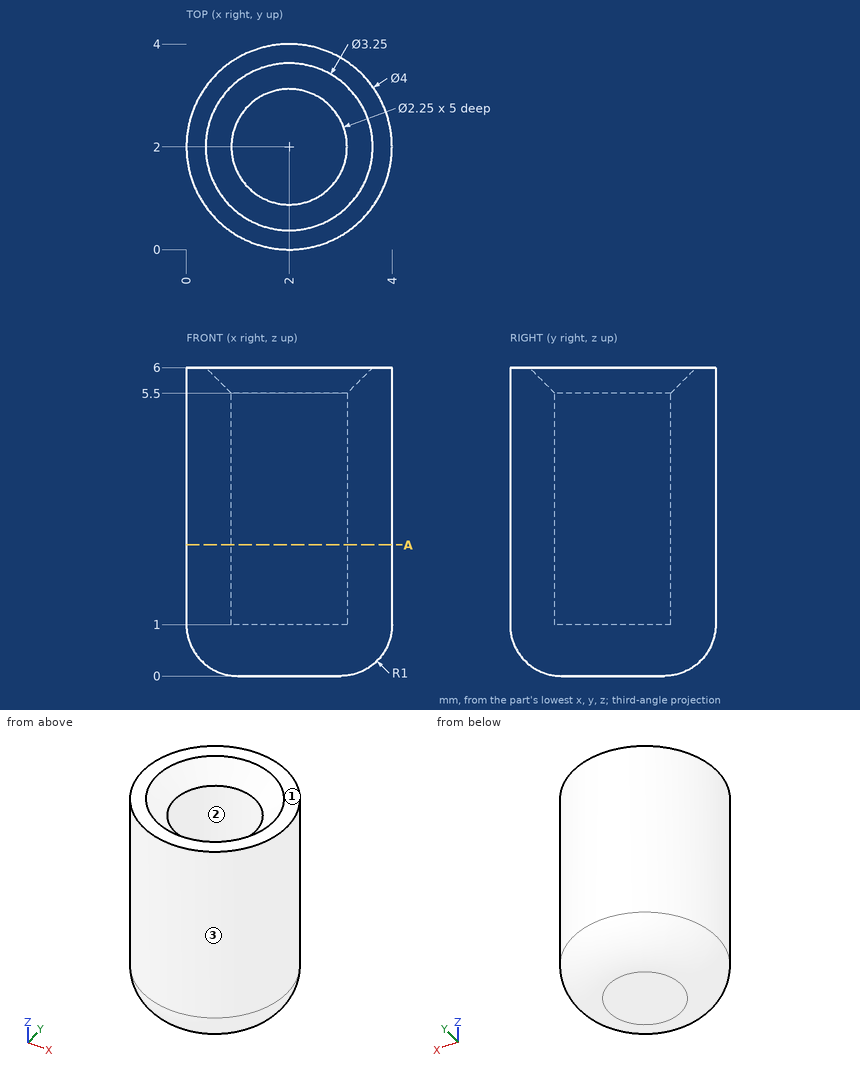
Part print with two shaded views. Sizes in mm from the minimum x, y, z corner. Coordinates: 2 decimals unless noted, no trailing zeros. Write each loop counter-clockwise with the first axis right and the second up, starting at its lowest first coordinate (ties: lowest second). Pieces come first, ordered by that corner, then holes. Notation, with made-up numbers: (70.25, 76.25) - (118.25, 76.25) arc R38 ccw to (118.25, 115.25) - close; hole circle Ø1 at (76, 43). An arc over 180 degrees is marked (long way). Use a Markdown table: item, result. Add a question column.
Item 1: Two-plate mould, pull along X, no slides. Class the marked faces 1, 2 and 3: pulls with the +X half, pulls with the -X half, needs draft (parallel to the pull), parting line crosses it, or undercut.
Item 2: Drop flat-ended pins along their axis: pin 1 (1 mm diameter, centred on x = 3, z = 3, fed in from +Y); pin 2 (1.1 mm diameter, centred on x = 2, y = 1.5, fed in from +Z). Give the stop position or say it passes through.
Item 3: Drill centre lines: line 1 along Y through (x, z) = (2, 3.65) (3 decimals); line 2 along Z through (x, y) = (1.75, 1.7); line 3 along X through (y, z) = (2.75, 2.05). Where is each one in solid material? Low to high.
Item 4: Band-saw the part on A-A, the plane z = 2.55. Write the cut outline in (x, y) (3 decimals).
A:
| question | item | result |
|---|---|---|
| 1 | face 1 | needs draft |
| 1 | face 2 | undercut |
| 1 | face 3 | parting line crosses it |
| 2 | pin 1 | stops at y = 3.94 |
| 2 | pin 2 | stops at z = 1 |
| 3 | line 1 | y = 0 to 0.875, 3.125 to 4 |
| 3 | line 2 | z = 0 to 1 |
| 3 | line 3 | x = 0.15 to 1.16, 2.84 to 3.85 |
| 4 | outline | circle Ø4 at (2, 2); hole circle Ø2.25 at (2, 2) |
